```python
from build123d import *

# Parameters (mm, degrees)
F0_W     = 457.2
F0_H     = 215.9
F0_W_2   = 25.4
F0_H_2   = 63.5
F0_W_3   = 19.05
F0_H_3   = 31.75
F0_W_4   = 12.7
F0_H_4   = 88.9
F0_W_5   = 53.975
F0_H_5   = 203.2
F0_H_6   = 25.4
F0_W_6   = 38.1
F0_W_7   = 28.575
F0_H_7   = 180.975
F0_H_8   = 161.925
F0_W_8   = 22.225
F0_W_9   = 22.86
F0_H_9   = 160.02
F1_DEPTH = 12.7
F2_W     = 457.2
F2_H     = 215.9
F3_DEPTH = 12.7


with BuildPart() as f1:
    # F0 (on Top) → F1 (new body)
    with BuildSketch(Plane.XY):
        with Locations((45.826613, -1.118122)):
            Rectangle(F0_W, F0_H)
        with Locations((-104.114569, -70.262038)):
            Rectangle(F0_W_2, F0_H_2, mode=Mode.SUBTRACT)
        with Locations((-100.939569, -14.362427)):
            Rectangle(F0_W_3, F0_H_3, mode=Mode.SUBTRACT)
        with Locations((142.704006, -13.470057)):
            Rectangle(F0_W_4, F0_H_4, mode=Mode.SUBTRACT)
        with Locations((-151.536249, -0.412038)):
            Rectangle(F0_W_5, F0_H_5, mode=Mode.SUBTRACT)
        with Locations((-100.939569, 21.679631)):
            Rectangle(F0_W_3, F0_H_6, mode=Mode.SUBTRACT)
        with Locations((-60.8544, -0.412038)):
            Rectangle(F0_W_6, F0_H_5, mode=Mode.SUBTRACT)
        with Locations((31.849021, 10.700462)):
            Rectangle(F0_W_7, F0_H_7, mode=Mode.SUBTRACT)
        with Locations((-9.525, 20.225462)):
            Rectangle(F0_W_3, F0_H_8, mode=Mode.SUBTRACT)
        with Locations((-102.527069, 53.399307)):
            Rectangle(F0_W_8, F0_H_6, mode=Mode.SUBTRACT)
        with Locations((78.221696, -0.978914)):
            Rectangle(F0_W_9, F0_H_9, mode=Mode.SUBTRACT)
    extrude(amount=F1_DEPTH)

    # F2 (on face) → F3 (join)
    with BuildSketch(Plane(origin=(0, 0, 0), x_dir=(1, 0, 0), z_dir=(0, 0, -1))):
        with Locations((45.826613, 1.118122)):
            Rectangle(F2_W, F2_H)
    extrude(amount=F3_DEPTH)


solid = f1.part
```
Verification items for the finished model (mm, model axes). A direction names the side the tool comes from. Coordinates: 2 decimals unless noted, no trailing zeros. Loops run counter-clockwise (first coordinate to the right, second up) from the corner with the lowest first, then second, coordinate; pieces in that order, holes last. Notation, with made-up numbers: (76, -3.5) -> (118, -3.5) arc R34 ccw to (118, 27.5) -> close; hole circle Ø7 at (43.25, 5.25). An arc over 180 degrees is marked (long way). Answer in a Markdown table with one row per item. Add a question column.
1. Section check C-C, the plane z = 4.25. Give the number of separate pieces and of enclosed holes in the cut face, then the cut area to 3 significant figures.
2. Draft check along X on faces 1 (the face through (-101, -15, 0)), 2 (the face through (43, -3, -12.7)), 3 (the face through (17.562, 9, 6)). Enter one of: +X half, -X half, draft (parallel to the pull), parting line (faces both ways), or undercut.
3. Section check A-A, the plane y = -70. Enter the section's corners in (x, z).
4. Access from +Z, -Z, +X, -X, +Y, -Y to the whole of each face (thin tool, end or side, straight path). Record for faces 4 (the face through (-110.465, 22, 6)), 5 (the face through (144, 48, 12.7)).
5. Material ranges on probe 1 along X at (y, z) = (89.5, 0.25); probe 2 along Y at (x, z) = (-47, 1); probe 3 along Y at (x, z) = (-0.5, 6.25), recorded low to high. Write a range as [from, to].
6. Section check B-B, the plane x = -101. Enter the section's corners in (y, z).
7. Depth check by flat-ended pin: P1, Ø9.5, axis at x = -8, y = 58.5, coming from the +Z side. Enter the tip coordinate at first touch or a pass-through.
Derived:
| question | item | result |
|---|---|---|
| 1 | separate pieces | 1 |
| 1 | enclosed holes | 10 |
| 1 | area | 63,700 mm² |
| 2 | face 1 | undercut |
| 2 | face 2 | draft |
| 2 | face 3 | undercut |
| 3 | outline | (-182.77, -12.7) -> (274.43, -12.7) -> (274.43, 12.7) -> (89.65, 12.7) -> (89.65, 0) -> (66.79, 0) -> (66.79, 12.7) -> (46.14, 12.7) -> (46.14, 0) -> (17.56, 0) -> (17.56, 12.7) -> (-41.8, 12.7) -> (-41.8, 0) -> (-79.9, 0) -> (-79.9, 12.7) -> (-91.41, 12.7) -> (-91.41, 0) -> (-116.81, 0) -> (-116.81, 12.7) -> (-124.55, 12.7) -> (-124.55, 0) -> (-178.52, 0) -> (-178.52, 12.7) -> (-182.77, 12.7) -> close |
| 4 | face 4 | +Z |
| 4 | face 5 | +Z, +X, -X, +Y, -Y |
| 5 | probe 1 | x = [-182.77, -178.52], [-124.55, -79.9], [-41.8, -19.05], [0, 17.56], [46.14, 274.43] |
| 5 | probe 2 | y = [-109.07, -102.01], [101.19, 106.83] |
| 5 | probe 3 | y = [-109.07, -60.74], [101.19, 106.83] |
| 6 | outline | (-109.07, -12.7) -> (106.83, -12.7) -> (106.83, 12.7) -> (66.1, 12.7) -> (66.1, 0) -> (40.7, 0) -> (40.7, 12.7) -> (34.38, 12.7) -> (34.38, 0) -> (8.98, 0) -> (8.98, 12.7) -> (1.51, 12.7) -> (1.51, 0) -> (-30.24, 0) -> (-30.24, 12.7) -> (-38.51, 12.7) -> (-38.51, 0) -> (-102.01, 0) -> (-102.01, 12.7) -> (-109.07, 12.7) -> close |
| 7 | P1 | stops at z = 0 |
